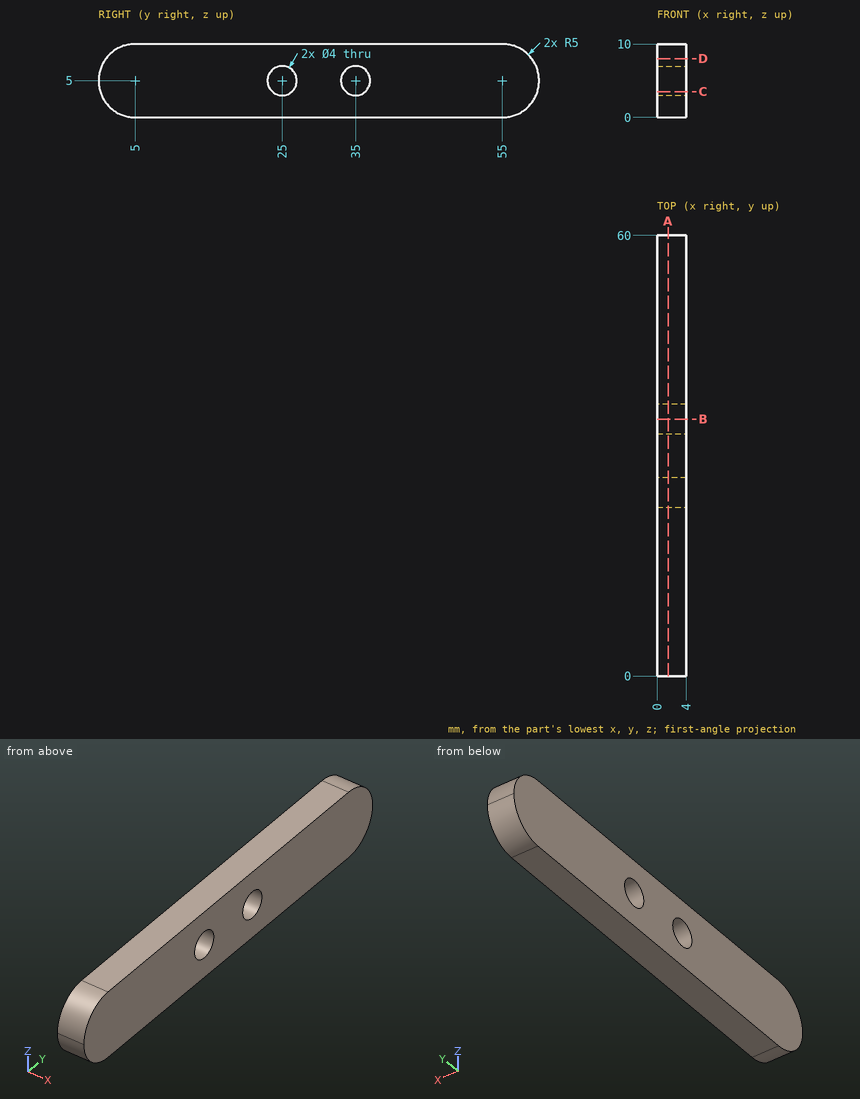
Verification items for this drawing (mm, ordinates from the low corner). Coordinates: 2 decimals unless noted, no trailing zeros. Order: outer loops, then holes, each group sorted by start corner. A loop starts at its lowest first (then second) coordinate and runs counter-clockwise, first axis right, second up. Notation, with made-up numbers: (-2, -9) - (21, -9) arc R6 cw to (21, -2) - close; hole circle Ø10 at (16, -22.5). An arc over 180 degrees is marked (long way). Use one line per item in the form item = value.
1. Section check A-A (x = 1.5). Record the boundary of the cut face in (y, z), then the cut area to 3 significant figures.
Here are the results:
outline = (0, 5) arc R5 ccw to (5, 0) - (55, 0) arc R5 ccw to (60, 5) arc R5 ccw to (55, 10) - (5, 10) arc R5 ccw to start; hole circle Ø4 at (25, 5); hole circle Ø4 at (35, 5)
area = 553 mm²
2. Section check B-B (y = 35). Record the boundary of the cut face in (x, z), then the cut area to 3 significant figures.
Here are the results:
outline = (0, 0) - (4, 0) - (4, 3) - (0, 3) - close; (0, 7) - (4, 7) - (4, 10) - (0, 10) - close
area = 24.0 mm²
3. Scan lines: line 1 (Z direction, x = 2.45, y = 25); line 2 (Y direction, x = 3.25, z = 6); line 3 (Y direction, x = 2.05, z = 7.25). Record each from-to range of solid material in increasing order.
Here are the results:
line_1 = 0 to 3, 7 to 10
line_2 = 0.1 to 23.27, 26.73 to 33.27, 36.73 to 59.9
line_3 = 0.53 to 59.47
4. Section check D-D (z = 8). Record the boundary of the cut face in (x, y), then the cut area to 3 significant figures.
Here are the results:
outline = (0, 1) - (4, 1) - (4, 59) - (0, 59) - close
area = 232 mm²
5. Section check C-C (z = 3.5). Record the boundary of the cut face in (x, y).
Here are the results:
outline = (0, 0.23) - (4, 0.23) - (4, 23.68) - (0, 23.68) - close; (0, 26.32) - (4, 26.32) - (4, 33.68) - (0, 33.68) - close; (0, 36.32) - (4, 36.32) - (4, 59.77) - (0, 59.77) - close
6. Gauge pin test, flat ends, axial feed: pin 1 (2.5 mm diameter, centred on y = 35, z = 5, fed in from -X); pin 2 (4.5 mm diameter, centred on y = 25, z = 5, fed in from -X). Record the tip position at first contact, or that the pin passes through.
Here are the results:
pin_1 = through
pin_2 = 0
